from build123d import *

# Parameters (mm, degrees)
SKETCH1_W           = 120
SKETCH1_H           = 120
BOSS_EXTRUDE1_DEPTH = 5
SKETCH2_R           = 2.5
CUT_EXTRUDE1_DEPTH  = 5
SKETCH3_R           = 2.5
CUT_EXTRUDE2_DEPTH  = 5
SKETCH4_R           = 2.5
CUT_EXTRUDE3_DEPTH  = 5
SKETCH5_R           = 2.5
CUT_EXTRUDE4_DEPTH  = 5
SKETCH6_W           = 10
SKETCH6_H           = 10
BOSS_EXTRUDE2_DEPTH = 10
SKETCH10_W          = 5
SKETCH10_H          = 5
BOSS_EXTRUDE4_DEPTH = 10
SKETCH11_W          = 5
SKETCH11_H          = 5
BOSS_EXTRUDE5_DEPTH = 10
SKETCH12_W          = 5
SKETCH12_H          = 5
BOSS_EXTRUDE6_DEPTH = 10
SKETCH13_W          = 5
SKETCH13_H          = 5
BOSS_EXTRUDE7_DEPTH = 10


with BuildPart() as part:
    # Sketch1 → Boss-Extrude1 (new body)
    with BuildSketch(Plane(origin=(0, 0, 0), x_dir=(1, 0, 0), z_dir=(0, 1, 0))):
        Rectangle(SKETCH1_W, SKETCH1_H)
    extrude(amount=BOSS_EXTRUDE1_DEPTH)

    # Sketch2 → Cut-Extrude1 (cut)
    with BuildSketch(Plane(origin=(0, 5, 0), x_dir=(1, 0, 0), z_dir=(0, 1, 0))):
        with Locations(Location((-25, 25, 0), (0, 0, 270))):
            Circle(SKETCH2_R)
    extrude(amount=-CUT_EXTRUDE1_DEPTH, mode=Mode.SUBTRACT)

    # Sketch3 → Cut-Extrude2 (cut)
    with BuildSketch(Plane(origin=(0, 5, 0), x_dir=(1, 0, 0), z_dir=(0, 1, 0))):
        with Locations(Location((25, 25, 0), (0, 0, 270))):
            Circle(SKETCH3_R)
    extrude(amount=-CUT_EXTRUDE2_DEPTH, mode=Mode.SUBTRACT)

    # Sketch4 → Cut-Extrude3 (cut)
    with BuildSketch(Plane(origin=(0, 5, 0), x_dir=(1, 0, 0), z_dir=(0, 1, 0))):
        with Locations(Location((25, -25, 0), (0, 0, 270))):
            Circle(SKETCH4_R)
    extrude(amount=-CUT_EXTRUDE3_DEPTH, mode=Mode.SUBTRACT)

    # Sketch5 → Cut-Extrude4 (cut)
    with BuildSketch(Plane(origin=(0, 5, 0), x_dir=(1, 0, 0), z_dir=(0, 1, 0))):
        with Locations(Location((-25, -25, 0), (0, 0, 270))):
            Circle(SKETCH5_R)
    extrude(amount=-CUT_EXTRUDE4_DEPTH, mode=Mode.SUBTRACT)

    # Sketch6 → Boss-Extrude2 (add)
    with BuildSketch(Plane(origin=(0, 5, 0), x_dir=(1, 0, 0), z_dir=(0, 1, 0))):
        Rectangle(SKETCH6_W, SKETCH6_H)
    extrude(amount=BOSS_EXTRUDE2_DEPTH)

    # Sketch10 → Boss-Extrude4 (add)
    with BuildSketch(Plane(origin=(0, 5, 0), x_dir=(1, 0, 0), z_dir=(0, 1, 0))):
        with Locations((42.5, 42.5)):
            Rectangle(SKETCH10_W, SKETCH10_H)
    extrude(amount=BOSS_EXTRUDE4_DEPTH)

    # Sketch11 → Boss-Extrude5 (add)
    with BuildSketch(Plane(origin=(0, 5, 0), x_dir=(1, 0, 0), z_dir=(0, 1, 0))):
        with Locations((-42.5, 42.5)):
            Rectangle(SKETCH11_W, SKETCH11_H)
    extrude(amount=BOSS_EXTRUDE5_DEPTH)

    # Sketch12 → Boss-Extrude6 (add)
    with BuildSketch(Plane(origin=(0, 5, 0), x_dir=(1, 0, 0), z_dir=(0, 1, 0))):
        with Locations((42.5, -42.5)):
            Rectangle(SKETCH12_W, SKETCH12_H)
    extrude(amount=BOSS_EXTRUDE6_DEPTH)

    # Sketch13 → Boss-Extrude7 (add)
    with BuildSketch(Plane(origin=(0, 5, 0), x_dir=(1, 0, 0), z_dir=(0, 1, 0))):
        with Locations((-42.5, -42.5)):
            Rectangle(SKETCH13_W, SKETCH13_H)
    extrude(amount=BOSS_EXTRUDE7_DEPTH)


solid = part.part
The listing builds one solid part. Answer for the finished solid, in the listing's coordinates (mm). A direction names the side the tool comes from. Coordinates: 2 decimals unless noted, no trailing zeros. Loops run counter-clockwise (first coordinate to the right, second up) from the corner with the lowest first, then second, coordinate; pieces in that order, holes last. Notation, with made-up numbers: M 78,60 L 113,60 A23 cw 113,86 Z; hole C 40,0 d10. An arc over 180 degrees is marked long. Answer in a Markdown table with one row per item.
1) Find section C-C (z = 25). Determine the outline of the cut face in (x, y), then the cut area to 3 significant figures.
Answers below:
| item | result |
|---|---|
| outline | M -60,0 L -27.5,0 L -27.5,5 L -60,5 Z; M -22.5,0 L 22.5,0 L 22.5,5 L -22.5,5 Z; M 27.5,0 L 60,0 L 60,5 L 27.5,5 Z |
| area | 550 mm^2 |
2) Given pin 1 (8 mm diameter, centred on y = 10.5, z = 0, fed in from +X); pin 2 (6 mm diameter, centred on x = -13.5, z = -29, fed in from +Y); pin 3 (3 mm diameter, centred on x = 2.5, y = 8, fed in from -Z), each flat-ended and moving along its own axis, determine where each tip first touches the part or whether it passes through.
Answers below:
| item | result |
|---|---|
| pin 1 | x = 5 |
| pin 2 | y = 5 |
| pin 3 | z = -5 |
3) Which of the six approach directions +Z, -Z, +X, -X, +Y, -Y give full straight-line access (tool end or side, diameter ignored) to faces 4 (the flat face through (-40, 10, 43)), 5 (the flat face through (0, 10, 5)), 6 (the flat face through (5, 10, 0))?
Answers below:
| item | result |
|---|---|
| face 4 | +Z, -Z, +Y |
| face 5 | +Z, +X, -X, +Y |
| face 6 | +Z, -Z, +X, +Y |
4) Determine the mould class of faces 1 (the flat face through (40, 10, -42)), 2 (the flat face through (-43, 10, -40)), 3 (the flat face through (-1, 2, -60)) for opening direction Z: released by +Z, released by -Z, zero draft, split by the parting line, or undercut.
Answers below:
| item | result |
|---|---|
| face 1 | zero draft |
| face 2 | undercut |
| face 3 | released by -Z |
5) Find section D-D (x = -1.5). Determine the outline of the cut face in (y, z), then the cut area to 3 significant figures.
Answers below:
| item | result |
|---|---|
| outline | M 0,-60 L 5,-60 L 5,-5 L 15,-5 L 15,5 L 5,5 L 5,60 L 0,60 Z |
| area | 700 mm^2 |
6) Find the intervals of material crossed by probe 1 along X at (y, z) = (1.45, 25); probe 2 along Z at (x, y) = (26.5, 3.5); probe 3 along X at (y, z) = (8.25, -43), in increasing order.
Answers below:
| item | result |
|---|---|
| probe 1 | -60 to -27.5, -22.5 to 22.5, 27.5 to 60 |
| probe 2 | -60 to -27, -23 to 23, 27 to 60 |
| probe 3 | -45 to -40, 40 to 45 |
7) Find section A-A (x = -25). Determine the outline of the cut face in (y, z).
Answers below:
| item | result |
|---|---|
| outline | M 0,-60 L 5,-60 L 5,-27.5 L 0,-27.5 Z; M 0,-22.5 L 5,-22.5 L 5,22.5 L 0,22.5 Z; M 0,27.5 L 5,27.5 L 5,60 L 0,60 Z |
8) Find section B-B (y = 12.75). Determine the outline of the cut face in (x, z), then the cut area to 3 significant figures.
Answers below:
| item | result |
|---|---|
| outline | M -45,-45 L -40,-45 L -40,-40 L -45,-40 Z; M -45,40 L -40,40 L -40,45 L -45,45 Z; M -5,-5 L 5,-5 L 5,5 L -5,5 Z; M 40,-45 L 45,-45 L 45,-40 L 40,-40 Z; M 40,40 L 45,40 L 45,45 L 40,45 Z |
| area | 200 mm^2 |
